```python
from build123d import *

# Parameters (mm, degrees)
SKETCH_1_W          = 9.5
SKETCH_1_H          = 0.5
SKETCH_2_R          = 2.5
CUT_EXTRUDE_1_DEPTH = 20.697715604


with BuildPart() as part:
    # 草图1 → 旋转1 (revolve)
    with BuildSketch(Plane.XY, mode=Mode.PRIVATE) as revolve_1_sk:
        Polygon((10, 5), (0, 5), (0, 0.25), (9.5, 0.25), (10, 0.25), (12, 2.25), (12, 3), align=None)
        Polygon((9.5, -0.25), (0, -0.25), (0, -5), (10, -5), (12, -3), (12, -2.25), (10, -0.25), align=None)
        with Locations((4.75, 0)):
            Rectangle(SKETCH_1_W, SKETCH_1_H)
    revolve(revolve_1_sk.sketch.rotate(Axis((0, 5, 0), (0, -1, 0)), 90), axis=Axis((0, 5, 0), (0, -1, 0)))

    # 草图2 → 切除-拉伸1 (cut, through all)
    with BuildSketch(Plane(origin=(0, 5, 0), x_dir=(1, 0, 0), z_dir=(0, 1, 0))):
        with Locations(Location((0, 0, 0), (0, 0, 270))):
            Circle(SKETCH_2_R)
    extrude(amount=-CUT_EXTRUDE_1_DEPTH, mode=Mode.SUBTRACT)


solid = part.part
```
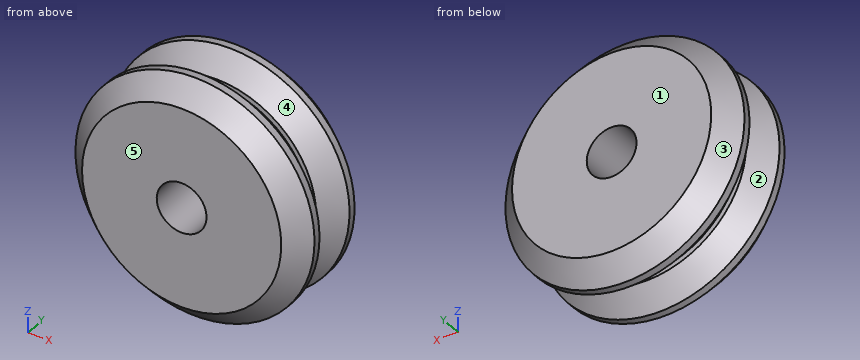
Model file for the job. Use its own axes, mm. Face numbers are marked on the shaded views. A direction names the side the tool comes from. Round coordinates to 2 decimals unless told otherwise and drop trailing zeros. Write each loop counter-clockwise with the first axis right and the second up, starting at its lowest first coordinate (ties: lowest second). Pieces come first, ordered by that corner, then holes. Notation, with made-up numbers: (80.5, 16.5) - (90.5, 16.5) arc R25 cw to (90.5, 51.5) - close; hole circle Ø2 at (-36.75, 23). An arc over 180 degrees is marked (long way). Use CSV: the item, a comma, the result in double quotes. Start each with the question number.
Item 1: Band-saw the part on D-D (y = 1.5). Write the cut outline in (x, z), and give its area (3 significant figures).
Item 2: Tool access for the marked faces 1 and 2: list every direction of +Z, -Z, +X, -X, +Y, -Y with a clear straight run to the whole face (end or side of a thin tool).
Item 3: Band-saw the part on B-B (x = 0). Write the cut outline in (y, z).
Item 4: Pin check, flat tips, straight feed: P1, Ø1, axis at y = -2.5, z = 7, coming from the -X side; P2, Ø5, axis at y = 2, z = -3, coming from the +X side; P3, Ø1.5, axis at x = 6.5, y = 3.5, coming from the -Z side. Stop position of each tip, or through.
Item 5: Drill centre lines: L1, parallel to Z at x = -1, y = -3.5; L2, parallel to Z at x = 1.5, y = 3.5; L3, parallel to X at y = -1, z = 0. Where is each one in solid material? Low to high. Write a range as [from, to].
Item 6: Two-plate mould, pull along Y, no slides. Class the marked faces 3, 4 and 5: released by +Y, released by -Y, zero draft, split by the parting line, or undercut.
Item 7: Band-saw the part on C-C (y = -3.5). Write the cut outline in (x, z), and give its area (3 significant figures).
Item 8: Band-saw the part on A-A (z = 0). Write the cut outline in (x, y), and give its area (4 significant figures).
Checked values:
1,outline,"circle Ø22.5 at (0, 0); hole circle Ø5 at (0, 0)"
1,area,"378 mm²"
2,face 1,"+Z, -Z, +X, -X, +Y"
2,face 2,"none"
3,outline,"(-5, -10) - (-3, -12) - (-2.25, -12) - (-0.25, -10) - (-0.25, -9.5) - (0.25, -9.5) - (0.25, -10) - (2.25, -12) - (3, -12) - (5, -10) - (5, -2.5) - (-5, -2.5) - close; (-5, 2.5) - (5, 2.5) - (5, 10) - (3, 12) - (2.25, 12) - (0.25, 10) - (0.25, 9.5) - (-0.25, 9.5) - (-0.25, 10) - (-2.25, 12) - (-3, 12) - (-5, 10) - close"
4,P1,"stops at x = -10.09"
4,P2,"stops at x = 11.99"
4,P3,"stops at z = -10.43"
5,L1,"z = [-11.46, -2.29], [2.29, 11.46]"
5,L2,"z = [-11.4, -2], [2, 11.4]"
5,L3,"x = [-10.75, -2.5], [2.5, 10.75]"
6,face 3,"released by +Y"
6,face 4,"undercut"
6,face 5,"released by -Y"
7,outline,"circle Ø23 at (0, 0); hole circle Ø5 at (0, 0)"
7,area,"396 mm²"
8,outline,"(-12, -3) - (-10, -5) - (-2.5, -5) - (-2.5, 5) - (-10, 5) - (-12, 3) - (-12, 2.25) - (-10, 0.25) - (-9.5, 0.25) - (-9.5, -0.25) - (-10, -0.25) - (-12, -2.25) - close; (2.5, -5) - (10, -5) - (12, -3) - (12, -2.25) - (10, -0.25) - (9.5, -0.25) - (9.5, 0.25) - (10, 0.25) - (12, 2.25) - (12, 3) - (10, 5) - (2.5, 5) - close"
8,area,"171.5 mm²"
